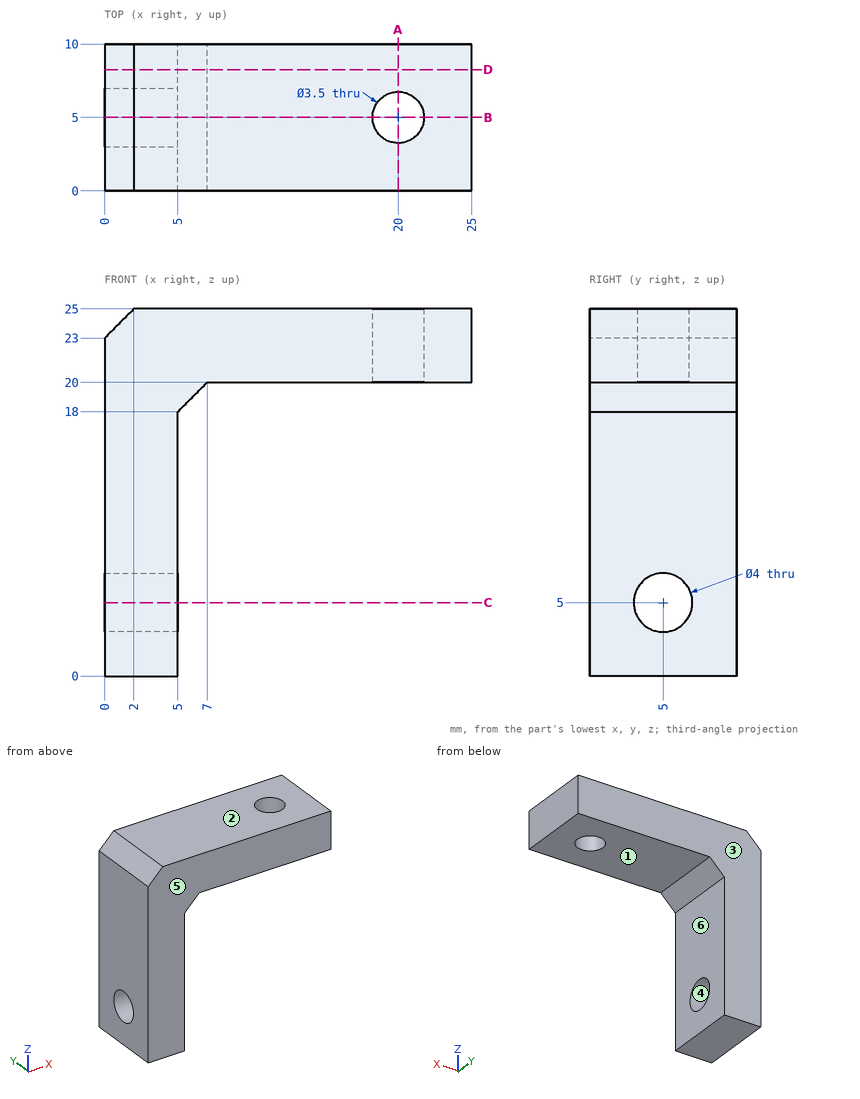
Answer from the drawing. Dimensions are ordinates in mm from the lowest x, y and z of the part. A direction names the side the tool comes from. Round coordinates to 2 decimals unless told otherwise and drop trailing zeros. Loops run counter-clockwise (first coordinate to the right, second up) from the corner with the lowest first, then second, coordinate; pieces in that order, holes last. Notation, with made-up numbers: (40.5, 74) - (69.5, 74) arc R25 ccw to (69.5, 98) - close; hole circle Ø2 at (-6.75, 83.5). An arc over 180 degrees is marked (long way). One line per item, written item: value.
Q1. Find section B-B on y = 5. Give the vertices of the cut face in (x, z), and give its area (4 significant figures).
Check values:
outline: (0, 0) - (5, 0) - (5, 3) - (0, 3) - close; (0, 7) - (5, 7) - (5, 18) - (7, 20) - (18.25, 20) - (18.25, 25) - (2, 25) - (0, 23) - close; (21.75, 20) - (25, 20) - (25, 25) - (21.75, 25) - close
area: 187.5 mm2
Q2. Straight lines are drawn through the part: probe 1 along Y at (x, z) = (1.55, 5); probe 2 along Y at (x, z) = (20, 21.15); probe 3 along Z at (x, y) = (13.25, 3). For each, find the intervals that lie inside material, in ascending order.
Check values:
probe 1: 0 to 3, 7 to 10
probe 2: 0 to 3.25, 6.75 to 10
probe 3: 20 to 25
Q3. Find section A-A on x = 20. Give the vertices of the cut face in (y, z).
Check values:
outline: (0, 20) - (3.25, 20) - (3.25, 25) - (0, 25) - close; (6.75, 20) - (10, 20) - (10, 25) - (6.75, 25) - close
Q4. Each of these flat-tipped pins is pushed along its axis until it touches: pin 1 Ø5 at (x, y) = (14, 5.5) entering from -Z; pin 2 Ø1.5 at (y, z) = (5, 11.5) entering from +X; pin 3 Ø8 at (x, z) = (11.5, 5) entering from -Y. Where does it stop, or does it pass through?
Check values:
pin 1: z = 20
pin 2: x = 5
pin 3: through
Q5. The mould has two halves that part along Z. Classify the marked faces 1, 2, 3 and 4: +Z half, -Z half, draft (parallel to the pull), parting line (faces both ways), or undercut.
Check values:
face 1: -Z half
face 2: +Z half
face 3: draft
face 4: undercut
Q6. For the marked faces 5 and 6, determine the directions among +Z, -Z, +X, -X, +Y, -Y from which every point of the face is accessible in a straight line to the end or side of a thin tool.
Check values:
face 5: +Z, -Z, +X, -X, -Y
face 6: -Z, +X, +Y, -Y
Q7. Find section C-C on z = 5. Give the vertices of the cut face in (x, y), and give its area (3 significant figures).
Check values:
outline: (0, 0) - (5, 0) - (5, 3) - (0, 3) - close; (0, 7) - (5, 7) - (5, 10) - (0, 10) - close
area: 30.0 mm2
Q8. Find section D-D on y = 8.25. Give the vertices of the cut face in (x, z), and give its area (3 significant figures).
Check values:
outline: (0, 0) - (5, 0) - (5, 18) - (7, 20) - (25, 20) - (25, 25) - (2, 25) - (0, 23) - close
area: 225 mm2
